Work out the finished part from the listing and answer in its coordinate system (mm). A direction names the side the tool comes from. Coordinates: 2 decimals unless noted, no trailing zeros. Write each loop counter-clockwise with the first axis right and the second up, starting at its lowest first coordinate (ties: lowest second). Pieces come first, ordered by that corner, then holes. Notation, with made-up numbers: M 23,73 L 48,73 A12 ccw 48,89 Z; hole C -20,54.25 d5. An arc over 180 degrees is marked long. Use CSV: the item, a comma, the result in double quotes.
from build123d import *

# Parameters (mm, degrees)
F1_DEPTH = 38.1


with BuildPart() as f1:
    # F0 (on Right) → F1 (new body)
    with BuildSketch(Plane.YZ):
        Polygon((-457.2, -304.8), (-457.2, -457.2), (-609.6, -457.2), (-609.6, -609.6), (-406.4, -609.6), (0, -203.2), (0, 0), (-152.4, 0), (-152.4, -152.4), (-304.8, -152.4), (-304.8, -304.8), align=None)
    extrude(amount=-F1_DEPTH)


solid = f1.part
Item 1: A tool of negligible diameter and unlimited length cuts with its end or side. For faces 1 (the face through (-19, -532, -457.2)), 2 (the face through (-19, 0, -103)), from which of +Z, -Z, +X, -X, +Y, -Y can it reach the whole face along a straight path? Write none if from no direction.
Answer:
face 1,"+Z, +X, -X, -Y"
face 2,"+Z, -Z, +X, -X, +Y"
Item 2: The part is cut by section A-A (x = -28.5). Write down the section's boundary in (y, z), then the cut area to 3 significant figures.
Answer:
outline,"M -609.6,-609.6 L -406.4,-609.6 L 0,-203.2 L 0,0 L -152.4,0 L -152.4,-152.4 L -304.8,-152.4 L -304.8,-304.8 L -457.2,-304.8 L -457.2,-457.2 L -609.6,-457.2 Z"
area,"150,000 mm2"
Item 3: Consider probe 1 along Y at (x, z) = (-18.5, -39.5); probe 2 along Z at (x, y) = (-23, -436.5); probe 3 along Z at (x, y) = (-16.5, -525). Determine where each line is inside the solid, lowest interval first.
Answer:
probe 1,"y = -152.4 to 0"
probe 2,"z = -609.6 to -304.8"
probe 3,"z = -609.6 to -457.2"
Item 4: Given pin 1 (8 mm diameter, centred on x = -15, z = -93, fed in from -Y); pin 2 (19 mm diameter, centred on x = -28, y = -523, fed in from +Z); pin 3 (12 mm diameter, centred on x = -18, z = -393, fed in from +Y), each flat-ended and moving along its own axis, determine where each tip first touches the part or whether it passes through.
Answer:
pin 1,"stops at y = -152.4"
pin 2,"stops at z = -457.2"
pin 3,"stops at y = -183.8"
Item 5: The part is cut by section B-B (y = -261). Write down the section's boundary in (x, z).
Answer:
outline,"M -38.1,-464.2 L 0,-464.2 L 0,-152.4 L -38.1,-152.4 Z"
Item 6: The part is cut by section C-C (z = -229.5). Write down the section's boundary in (x, y).
Answer:
outline,"M -38.1,-304.8 L 0,-304.8 L 0,-26.3 L -38.1,-26.3 Z"
